```python
from build123d import *

# Parameters (mm, degrees)
SKETCH_1_R           = 35.5
SKETCH_1_R_2         = 2
EXTRUDE_4_DEPTH      = 10
SKETCH_24_W          = 98
SKETCH_24_H          = 6
EXTRUDE_5_DEPTH      = 3
SKETCH_26_W          = 98
SKETCH_26_H          = 35
CUT_EXTRUDE_17_DEPTH = 7
CHAMFER_1_SIZE       = 7
SKETCH_27_R          = 3.1
CUT_EXTRUDE_18_DEPTH = 5
SKETCH_28_R          = 2
CUT_EXTRUDE_19_DEPTH = 15


with BuildPart() as part:
    # 스케치1 → 보스-돌출4 (new body)
    with BuildSketch(Plane(origin=(0, 0, 0), x_dir=(1, 0, 0), z_dir=(0, 1, 0))):
        with BuildLine():
            Line((-49, 0), (-49, -53))
            Line((-49, -53), (49, -53))
            Line((49, -53), (49, 0))
            ThreePointArc((49, 0), (0, 49), (-49, 0))
        make_face()
        with Locations(Location((0, 0, 0), (0, 0, 270))):
            Circle(SKETCH_1_R, mode=Mode.SUBTRACT)
        with Locations(Location((-43.466662183, 11.64685703, 0), (0, 0, 270))):
            Circle(SKETCH_1_R_2, mode=Mode.SUBTRACT)
        with Locations(Location((-11.64685703, 43.466662183, 0), (0, 0, 270))):
            Circle(SKETCH_1_R_2, mode=Mode.SUBTRACT)
        with Locations(Location((31.819805153, 31.819805153, 0), (0, 0, 270))):
            Circle(SKETCH_1_R_2, mode=Mode.SUBTRACT)
        with Locations(Location((43.466662183, -11.64685703, 0), (0, 0, 270))):
            Circle(SKETCH_1_R_2, mode=Mode.SUBTRACT)
        with Locations(Location((11.64685703, -43.466662183, 0), (0, 0, 270))):
            Circle(SKETCH_1_R_2, mode=Mode.SUBTRACT)
        with Locations(Location((-31.819805153, -31.819805153, 0), (0, 0, 270))):
            Circle(SKETCH_1_R_2, mode=Mode.SUBTRACT)
    extrude(amount=EXTRUDE_4_DEPTH)

    # 스케치24 → 보스-돌출5 (add)
    with BuildSketch(Plane.XY.offset(53)):
        with Locations((0, 5)):
            Rectangle(SKETCH_24_W, SKETCH_24_H)
    extrude(amount=EXTRUDE_5_DEPTH)

    # 스케치26 → 컷-돌출17 (cut)
    with BuildSketch(Plane(origin=(0, 10, 0), x_dir=(1, 0, 0), z_dir=(0, 1, 0))):
        Rectangle(SKETCH_26_W, SKETCH_26_H)
    extrude(amount=-CUT_EXTRUDE_17_DEPTH, mode=Mode.SUBTRACT)

    # 모따기1
    chamfer_1_edges = [part.edges().sort_by_distance(p)[0] for p in [
        (-39.943445211, 10, 17.5),
        (39.943445211, 10, 17.5),
        (38.327664665, 10, -17.5),
        (-38.327664665, 10, -17.5),
    ]]
    chamfer(chamfer_1_edges, length=CHAMFER_1_SIZE - 0.0001)  # a hair under: the kernel refuses the full size

    # 스케치27 → 컷-돌출18 (cut)
    with BuildSketch(Plane(origin=(0, 10, 0), x_dir=(1, 0, 0), z_dir=(0, 1, 0))):
        with Locations(Location((-11.64685703, 43.466662183, 0), (0, 0, 270))):
            Circle(SKETCH_27_R)
        with Locations(Location((31.819805153, 31.819805153, 0), (0, 0, 270))):
            Circle(SKETCH_27_R)
        with Locations((43.466662183, -11.64685703)):
            Circle(SKETCH_27_R)
        with Locations(Location((11.64685703, -43.466662183, 0), (0, 0, 270))):
            Circle(SKETCH_27_R)
        with Locations(Location((-31.819805153, -31.819805153, 0), (0, 0, 270))):
            Circle(SKETCH_27_R)
        with Locations((-43.466662183, 11.64685703)):
            Circle(SKETCH_27_R)
    extrude(amount=-CUT_EXTRUDE_18_DEPTH, mode=Mode.SUBTRACT)

    # 스케치28 → 컷-돌출19 (cut)
    with BuildSketch(Plane.XY.offset(56)):
        with Locations((-36, 5)):
            Circle(SKETCH_28_R)
        with Locations((-18, 5)):
            Circle(SKETCH_28_R)
        with Locations((0, 5)):
            Circle(SKETCH_28_R)
        with Locations((18, 5)):
            Circle(SKETCH_28_R)
        with Locations((36, 5)):
            Circle(SKETCH_28_R)
    extrude(amount=-CUT_EXTRUDE_19_DEPTH, mode=Mode.SUBTRACT)


solid = part.part
```
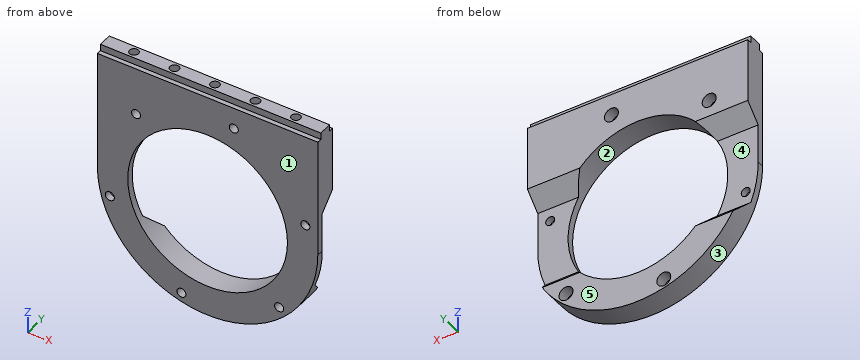
Verification items for the finished model (mm, model axes). Face numbers are marked on the shaded views. A direction names the side the tool comes from. Coordinates: 2 decimals unless noted, no trailing zeros. Order: outer loops, then holes, each group sorted by start corner. A loop starts at its lowest first (then second) coordinate and runs counter-clockwise, first axis right, second up. Notation, with made-up numbers: (-18.75, 83.5) -> (-3.75, 83.5) arc R17 ccw to (-3.75, 96.5) -> close; hole circle Ø11 at (-12, -10). An arc over 180 degrees is marked (long way). Answer as CSV lines item,"result". Start each with the question number.
1) Cross-section at C-C, the plane x = 18. Record the boundary of the cut face in (y, z).
2) Set-up check for the marked faces 4 and 5: record each of +Z, -Z, +X, -X, +Y, -Y from which the full face is reachable in a straight line by a thin tool's end or side.
3) Cross-section at A-A, the plane z = -23. Record the boundary of the cut face in (x, y).
4) Cross-section at B-B, the plane z = 43. Record the boundary of the cut face in (x, y).
5) Gauge pin test, flat ends, axial feed: pin 1 Ø1.2 at (x, y) = (18.5, 5) entering from +Z; pin 2 Ø1 at (x, y) = (3, 0.5) entering from +Z; pin 3 Ø0.9 at (x, z) = (24, 55) entering from -Y. Record the tip position at first contact, or that the pin passes through.
6) Cross-section at D-D, the plane z = -6.5. Record the boundary of the cut face in (x, y).
7) Release check for a two-part mould opening along Z. For the marked faces 1, 2 and 3 record: released by +Z, released by -Z, zero draft, split by the parting line, or undercut.
8) Material ranges on L1, parallel to Z at x = -11, y = 2.5; L2, parallel to Y at x = -13, z = -41.5; L3, parallel to X at y = 4.5, z = 32.5, recorded low to high. Write a range as [from, to].
Conclusion:
1,outline,"(0, -45.57) -> (10, -45.57) -> (10, -30.6) -> (0, -30.6) -> close; (0, 30.6) -> (10, 30.6) -> (10, 53) -> (8, 53) -> (8, 56) -> (7, 56) -> (7, 41) -> (3, 41) -> (3, 56) -> (2, 56) -> (2, 53) -> (0, 53) -> close"
2,face 4,"+X, -X, +Y"
2,face 5,"+Z, -Z, +X, -X, +Y"
3,outline,"(-43.27, 0) -> (-27.04, 0) -> (-27.04, 8.5) -> (-43.27, 8.5) -> close; (27.04, 0) -> (43.27, 0) -> (43.27, 8.5) -> (27.04, 8.5) -> close"
4,outline,"(-49, 0) -> (9.7, 0) -> (9.7, 5) -> (8.58, 5) -> (8.58, 10) -> (-49, 10) -> close; (13.59, 0) -> (49, 0) -> (49, 10) -> (14.71, 10) -> (14.71, 5) -> (13.59, 5) -> close; hole circle Ø4 at (-36, 5); hole circle Ø4 at (-18, 5); hole circle Ø4 at (0, 5); hole circle Ø4 at (18, 5); hole circle Ø4 at (36, 5)"
5,pin 1,"stops at z = 41"
5,pin 2,"stops at z = 53"
5,pin 3,"stops at y = 2"
6,outline,"(-48.57, 0) -> (-34.9, 0) -> (-34.9, 3) -> (-48.57, 3) -> close; (34.9, 0) -> (48.57, 0) -> (48.57, 3) -> (34.9, 3) -> close"
7,face 1,"zero draft"
7,face 2,"undercut"
7,face 3,"released by -Z"
8,L1,"z = [-47.75, -45.36], [-41.57, -33.75], [33.75, 56]"
8,L2,"y = [0, 5]"
8,L3,"x = [-49, -33.7], [-29.94, -14.28], [14.28, 49]"
